CAD build for the part. Positions are in the model's coordinates, mm. Round coordinates to 2 decimals unless told otherwise and drop trailing zeros. Loops run counter-clockwise (first coordinate to the right, second up) from the corner with the lowest first, then second, coordinate; pieces in that order, holes last. Notation, with made-up numbers: (23, -5.75) - (76, -5.75) arc R12 cw to (76, 5.25) - close; hole circle Ø7 at (27.5, 76). An arc over 180 degrees is marked (long way). Use one line per item in the form item = value.
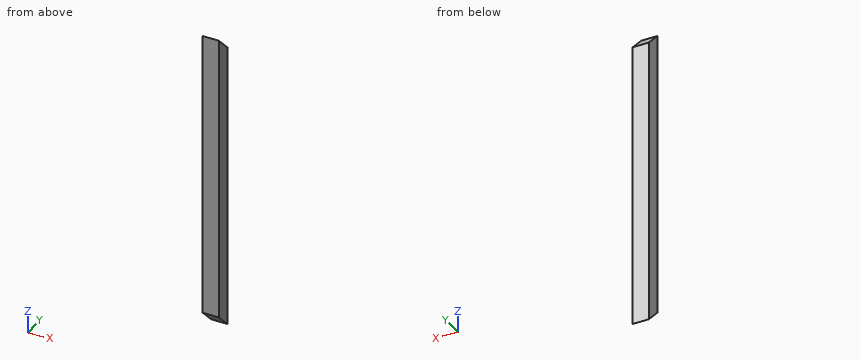
from build123d import *

# Parameters (mm, degrees)
F0_W          = 50
F0_H          = 50
F1_DEPTH      = 950
F3_DEPTH      = 25.001
F3_DEPTH_BACK = 25.001
F5_DEPTH      = 25.001
F5_DEPTH_BACK = 25.001


with BuildPart() as f1:
    # F0 (on Top) → F1 (new body)
    with BuildSketch(Plane.XY):
        Rectangle(F0_W, F0_H)
    extrude(amount=F1_DEPTH)

    # F2 (on Right) → F3 (cut, two sides)
    with BuildSketch(Plane.YZ) as f3_sk:
        Polygon((135.3058686236, 950), (-25, 950), (135.3058686236, 789.6941313764), align=None)
    extrude(amount=-F3_DEPTH, mode=Mode.SUBTRACT)
    extrude(f3_sk.sketch, amount=F3_DEPTH_BACK, mode=Mode.SUBTRACT)

    # F4 (on Right) → F5 (cut, two sides)
    with BuildSketch(Plane.YZ) as f5_sk:
        Polygon((-25, 0), (25, 0), (-25, 50), align=None)
    extrude(amount=-F5_DEPTH, mode=Mode.SUBTRACT)
    extrude(f5_sk.sketch, amount=F5_DEPTH_BACK, mode=Mode.SUBTRACT)


solid = f1.part
1) Drill centre lines: probe 1 along Z at (x, y) = (2, 17); probe 2 along Z at (x, y) = (15.5, -8.5). Where is each one in solid material? Low to high.
Report:
probe_1 = 8 to 908
probe_2 = 33.5 to 933.5
2) Slice it at A-A (x = 1). Write the cut outline in (y, z).
Report:
outline = (-25, 50) - (25, 0) - (25, 900) - (-25, 950) - close
3) Slice it at B-B (y = -0.5). Write the cut outline in (x, z), plus the area to 3 significant figures.
Report:
outline = (-25, 25.5) - (25, 25.5) - (25, 925.5) - (-25, 925.5) - close
area = 45,000 mm^2
4) Flat gauge pins, fed straight in: pin 1 (6 mm diameter, centred on x = 12, y = -16, fed in from +Z); pin 2 (1.5 mm diameter, centred on x = 9.5, y = -12, fed in from -Z); pin 3 (5 mm diameter, centred on x = 15, y = -2, fed in from -Z). Where does each tip first touch, or does it go through?
Report:
pin_1 = 944
pin_2 = 36.25
pin_3 = 24.5
